Can you work these out from the model? Positions are in its coordinate system, mm. A direction names the side the tool comes from. Coordinates: 2 decimals unless noted, no trailing zeros. Order: outer loops, then holes, each group sorted by start corner. A loop starts at its lowest first (then second) coordinate and runs counter-clockwise, first axis right, second up. Notation, with made-up numbers: (-10, 30.5) -> (7, 30.5) arc R15 ccw to (7, 38.5) -> close; hole circle Ø1 at (54.25, 47). An arc over 180 degrees is marked (long way). Use a Markdown table: item, result. Add a question column.
1. If I drill on line 1 along Y through (x, z) = (-10.5, 2.05); line 2 along X through (y, z) = (11, 1.45); line 3 along X through (y, z) = (8, 1.45), over which ranges is the centre line in solid material (lowest first)? Write a range as from..to.
2. We'd pull the mould along X, two halves only. Please class faces 1 (the cylindrical face through (-0.857, 20.982, 1.717)), 2 (the flat face through (4.11, -18.91, 1.72)), 3 (the flat face through (1.7, 17.3, 1.15)): pulls with the +X half, pulls with the -X half, needs draft (parallel to the pull), parting line crosses it, or undercut.
3. Suppose I cut it at D-D, the plane z = 1.5. List the corners of the cut face in (x, y) for me (1 decimal).
4. For pin 1 Ø3 at (x, y) = (-5.97, -16.41) entering from -Z, with a flat end and sliding along its axis, tell me the tip position at first contact or that it passes through.
5. Suppose I cut it at B-B, the plane y = 0. List the corners of the cut face in (x, z) for me.
6. Suppose I cut it at A-A, the plane x = -6.5. List the corners of the cut face in (y, z) for me.
7. Suppose I cut it at C-C, the plane x = 18. List the corners of the cut face in (y, z) for me.
8. For faces 4 (the cylindrical face through (-7.006, -17.2, 1.717)), 5 (the flat face through (-4.09, -18.86, 1.72)), which set-ups out of +Z, -Z, +X, -X, +Y, -Y let a thin tool reach every point of the face, with its end or its side?
```python
from build123d import *
from build123d.topology import SkipClean

# Parameters (mm, degrees)
SKETCH1_R                 = 21
EXTRUDE1_DEPTH            = 1.15
SKETCH34_R                = 1.303333333
F_056_250_SNAP_RING_DEPTH = 1.15
SKETCH35_R                = 21
CUT_EXTRUDE1_DEPTH        = 1.15


with BuildPart() as part:
    # Sketch1 → Extrude1 (new body)
    with BuildSketch(Plane.XY):
        Circle(SKETCH1_R)
    extrude(amount=EXTRUDE1_DEPTH)

    # Sketch34 → 056-250 Snap Ring (add)
    with SkipClean():  # the faces are left unmerged after this step: merging them gives an invalid solid
        with BuildSketch(Plane.XY.offset(1.15)):
            with BuildLine():
                Line((-3.522256245, -17.298702968), (-4.677411169, -20.472465039))
                ThreePointArc((-4.677411169, -20.472465039), (0, 21), (4.677411169, -20.472465039))
                Line((4.677411169, -20.472465039), (3.522256245, -17.298702968))
                ThreePointArc((3.522256245, -17.298702968), (4.842117839, -14.057977774), (8.197569602, -15.050589419))
                ThreePointArc((8.197569602, -15.050589419), (10.018304079, -16.269002398), (12.125199981, -15.668507704))
                ThreePointArc((12.125199981, -15.668507704), (0, 16.9723), (-12.125199981, -15.668507704))
                ThreePointArc((-12.125199981, -15.668507704), (-10.018304079, -16.269002398), (-8.197569602, -15.050589419))
                ThreePointArc((-8.197569602, -15.050589419), (-4.842117839, -14.057977774), (-3.522256245, -17.298702968))
            make_face()
            with Locations((5.971721676, -16.407170461)):
                Circle(SKETCH34_R, mode=Mode.SUBTRACT)
            with Locations((-5.971721676, -16.407170461)):
                Circle(SKETCH34_R, mode=Mode.SUBTRACT)
        extrude(amount=F_056_250_SNAP_RING_DEPTH)

    # Sketch35 → Cut-Extrude1 (cut)
    with BuildSketch(Plane(origin=(0, 0, 0), x_dir=(-1, 0, 0), z_dir=(0, 0, -1))):
        Circle(SKETCH35_R)
    extrude(amount=-CUT_EXTRUDE1_DEPTH, mode=Mode.SUBTRACT)


solid = part.part
```
Worked out:
| question | item | result |
|---|---|---|
| 1 | line 1 | y = -18.19..-16.3, 13.72..18.19 |
| 1 | line 2 | x = -17.89..-13.64, 13.64..17.89 |
| 1 | line 3 | x = -19.42..-15.9, 15.9..19.42 |
| 2 | face 1 | parting line crosses it |
| 2 | face 2 | undercut |
| 2 | face 3 | needs draft |
| 3 | outline | (-12.1, -15.7) arc R18.6 cw (long way) to (12.1, -15.7) arc R2.6 cw to (8.2, -15.1) arc R2.6 ccw to (3.5, -17.3) -> (4.7, -20.5) arc R21 ccw (long way) to (-4.7, -20.5) -> (-3.5, -17.3) arc R2.6 ccw to (-8.2, -15.1) arc R2.6 cw to start; hole circle Ø2.6 at (-6, -16.4); hole circle Ø2.6 at (6, -16.4) |
| 4 | pin 1 | stops at z = 1.15 |
| 5 | outline | (-21, 1.15) -> (-18.5, 1.15) -> (-18.5, 2.3) -> (-21, 2.3) -> close; (18.5, 1.15) -> (21, 1.15) -> (21, 2.3) -> (18.5, 2.3) -> close |
| 6 | outline | (-19.97, 1.15) -> (-17.6, 1.15) -> (-17.6, 2.3) -> (-19.97, 2.3) -> close; (-15.22, 1.15) -> (-13.85, 1.15) -> (-13.85, 2.3) -> (-15.22, 2.3) -> close; (15.8, 1.15) -> (19.97, 1.15) -> (19.97, 2.3) -> (15.8, 2.3) -> close |
| 7 | outline | (-10.82, 1.15) -> (-6.18, 1.15) -> (-6.18, 2.3) -> (-10.82, 2.3) -> close; (2.98, 1.15) -> (10.82, 1.15) -> (10.82, 2.3) -> (2.98, 2.3) -> close |
| 8 | face 4 | +Z, -Z |
| 8 | face 5 | +Z, -Z, -Y |
